Can you work these out from the model? Positions are in its coordinate system, mm. Coordinates: 2 decimals unless noted, no trailing zeros. Loops run counter-clockwise (first coordinate to the right, second up) from the corner with the lowest first, then second, coordinate; pieces in that order, holes last. Notation, with made-up numbers: M -23.5,-16.75 L 35.5,-16.75 A30 cw 35.5,8.25 Z; hole C 14.25,56.5 d11. An arc over 180 degrees is marked long. Return JSON: item names as keys, results as strings. Group by question number.
Autodesk Inventor part; units mm, degrees
ref_plane "YZ Plane" through (0, 0, 0) normal (1, 0, 0) x (0, 1, 0)
ref_plane "XZ Plane" through (0, 0, 0) normal (0, 1, 0) x (-1, 0, 0)
ref_plane "XY Plane" through (0, 0, 0) normal (0, 0, 1) x (1, 0, 0)
sketch "Sketch1" plane through (0, 0, 0) normal (1, 0, 0) x (0, 1, 0)
  line L0 (-50, 50) -> (50, 50)
  line L1 (50, 50) -> (50, -50)
  line L2 (50, -50) -> (-50, -50)
  line L3 (-50, -50) -> (-50, 50)
  line L4 (-50, 50) -> (50, -50) construction
  line L5 (50, 50) -> (-50, -50) construction
  line L6 (50, 50) -> (-50, 50)
  line L7 (-50, 50) -> (-50, 310)
  line L8 (-50, 310) -> (50, 310)
  line L9 (50, 310) -> (50, 50)
  line L10 (50, -50) -> (-50, -50)
  line L11 (-50, -50) -> (-50, -310)
  line L12 (-50, -310) -> (50, -310)
  line L13 (50, -310) -> (50, -50)
  line L14 (-50, 255) -> (-55, 255)
  line L15 (-55, 255) -> (-55, 205)
  line L16 (-55, 205) -> (-50, 205)
  line L17 (-50, 205) -> (-50, 255)
  line L18 (-50, 155) -> (-55, 155)
  line L19 (-55, 155) -> (-55, 105)
  line L20 (-55, 105) -> (-50, 105)
  line L21 (-50, 105) -> (-50, 155)
  line L22 (-50, 25) -> (-55, 25)
  line L23 (-55, 25) -> (-55, -25)
  line L24 (-55, -25) -> (-50, -25)
  line L25 (-50, -25) -> (-50, 25)
  line L26 (-50, -105) -> (-55, -105)
  line L27 (-55, -105) -> (-55, -155)
  line L28 (-55, -155) -> (-50, -155)
  line L29 (-50, -155) -> (-50, -105)
  line L30 (-50, -205) -> (-55, -205)
  line L31 (-55, -205) -> (-55, -255)
  line L32 (-55, -255) -> (-50, -255)
  line L33 (-50, -255) -> (-50, -205)
  line L34 (50, 310) -> (30, 310)
  line L35 (50, 305) -> (50, 310)
  line L36 (-50, 310) -> (-30, 310)
  line L37 (-50, 305) -> (-50, 310)
  line L38 (30, 50) -> (-30, 50)
  line L39 (-30, 50) -> (-30, 55)
  line L40 (-30, 55) -> (30, 55)
  line L41 (30, 55) -> (30, 50)
  line L42 (30, -50) -> (-36.1124, -50)
  line L43 (50, 0) -> (-50, 0) construction
  line L44 (-30, -50) -> (-30, -55)
  line L45 (-30, -55) -> (30, -55)
  line L46 (30, -55) -> (30, -50)
  line L47 (30, 310) -> (-30, 310)
  line L48 (-30, 310) -> (-30, 305)
  line L49 (-30, 305) -> (30, 305)
  line L50 (30, 305) -> (30, 310)
  line L51 (-30, -310) -> (-30, -305)
  line L52 (-30, -305) -> (30, -305)
  line L53 (30, -305) -> (30, -310)
  line L54 (-50, -180) -> (50, -180) construction
  circle A0 centre (0, -180) radius 16
  line L55 (50, 25) -> (45, 25)
  line L56 (45, 25) -> (45, -25)
  line L57 (45, -25) -> (50, -25)
  line L58 (50, -25) -> (50, 25)
  line L59 (50, -105) -> (45, -105)
  line L60 (45, -105) -> (45, -155)
  line L61 (45, -155) -> (50, -155)
  line L62 (50, -155) -> (50, -105)
  line L63 (50, -255) -> (45, -255)
  line L64 (45, -255) -> (45, -205)
  line L65 (45, -205) -> (50, -205)
  line L66 (-50, 11.5) -> (-32, 11.5)
  line L67 (-32, 11.5) -> (-32, -11.5)
  line L68 (-32, -11.5) -> (-50, -11.5)
  line L69 (-50, -11.5) -> (-50, 11.5)
  line L70 (-33.6603, 235) -> (-25, 240)
  line L71 (-25, 240) -> (-16.3397, 235)
  line L72 (-16.3397, 235) -> (-16.3397, 225)
  line L73 (-16.3397, 225) -> (-25, 220)
  line L74 (-25, 220) -> (-33.6603, 225)
  line L75 (-33.6603, 225) -> (-33.6603, 235)
  line L76 (-33.6603, 135) -> (-25, 140)
  line L77 (-25, 140) -> (-16.3397, 135)
  line L78 (-16.3397, 135) -> (-16.3397, 125)
  line L79 (-16.3397, 125) -> (-25, 120)
  line L80 (-25, 120) -> (-33.6603, 125)
  line L81 (-33.6603, 125) -> (-33.6603, 135)
  line L82 (-8.75, 225) -> (-13.75, 225)
  line L83 (-13.75, 225) -> (-13.75, 205)
  line L84 (-13.75, 205) -> (-8.75, 205)
  line L85 (-8.75, 205) -> (-8.75, 225)
  line L86 (-13.75, 135) -> (-8.75, 135)
  line L87 (-8.75, 135) -> (-8.75, 155)
  line L88 (-8.75, 155) -> (-13.75, 155)
  line L89 (-13.75, 155) -> (-13.75, 135)
  line L90 (-13.75, 85) -> (-8.75, 85)
  line L91 (-8.75, 85) -> (-8.75, 65)
  line L92 (-8.75, 65) -> (-13.75, 65)
  line L93 (-13.75, 65) -> (-13.75, 85)
  line L94 (-25, 314.14) -> (-25, -94.5604) construction
  line L95 (-41.25, 225) -> (-36.25, 225)
  line L96 (-36.25, 225) -> (-36.25, 205)
  line L97 (-36.25, 205) -> (-41.25, 205)
  line L98 (-41.25, 205) -> (-41.25, 225)
  line L99 (-36.25, 135) -> (-41.25, 135)
  line L100 (-41.25, 135) -> (-41.25, 155)
  line L101 (-41.25, 155) -> (-36.25, 155)
  line L102 (-36.25, 155) -> (-36.25, 135)
  line L103 (-36.25, 85) -> (-41.25, 85)
  line L104 (-41.25, 85) -> (-41.25, 65)
  line L105 (-41.25, 65) -> (-36.25, 65)
  line L106 (-36.25, 65) -> (-36.25, 85)
  line L107 (-15, 242.5) -> (-35, 242.5)
  line L108 (-35, 242.5) -> (-35, 247.5)
  line L109 (-35, 247.5) -> (-15, 247.5)
  line L110 (-15, 247.5) -> (-15, 242.5)
  line L111 (-15, 20) -> (-35, 20)
  line L112 (-35, 20) -> (-35, 25)
  line L113 (-35, 25) -> (-15, 25)
  line L114 (-15, 25) -> (-15, 20)
  line L115 (-20, 42.5) -> (-30, 42.5)
  line L116 (-30, 42.5) -> (-30, 32.5)
  line L117 (-30, 32.5) -> (-20, 32.5)
  line L118 (-20, 32.5) -> (-20, 42.5)
  point P0 (0, 0)
  point P1 (-52.5, 155)
  point P2 (-52.5, 205)
  point P3 (-50, 205)
  point P4 (-50, 105)
  point P5 (-50, -155)
  point P6 (-50, -255)
  point P7 (30, -50)
  point P8 (-30, -50)
  point P9 (-30, 50)
  point P10 (30, 50)
  point P11 (30, 307.5)
  point P12 (-30, -310)
  point P13 (30, -310)
  point P14 (30, 310)
  point P15 (-30, 310)
  point P16 (50, -25)
  point P17 (50, -255)
  point P18 (50, -205)
  point P19 (50, -155)
  point P20 (-50, 0)
  point P21 (-50, 11.5)
  point P22 (-50, -11.5)
  point P23 (-25, 230)
  point P24 (-25, 130)
  point P25 (-13.75, 145)
  point P26 (-36.25, 145)
  point P27 (-15, 22.5)
  point P28 (-30, 37.5)
  dimension "d0" = 100
  dimension "d1" = 260
  dimension "d2" = 100
  dimension "d3" = 260
  dimension "d4" = 50
  dimension "d5" = 50
  dimension "d6" = 50
  dimension "d7" = 50
  dimension "d8" = 50
  dimension "d9" = 55
  dimension "d10" = 50
  dimension "d11" = 25
  dimension "d12" = 55
  dimension "d13" = 50
  dimension "d14" = 5
  dimension "d20" = 5
  dimension "d21" = 5
  dimension "d23" = 20
  dimension "d26" = 32
  dimension "d27" = 5
  dimension "d28" = 5
  dimension "d29" = 18
  dimension "d30" = 23
  dimension "d31" = 11.5
  dimension "d32" = 20
  dimension "d34" = 10
  dimension "d35" = 25
  dimension "d37" = 25
  dimension "d38" = 16.3397
  dimension "d39" = 10
  dimension "d40" = 25
  dimension "d41" = 16.3397
  dimension "d42" = 25
  dimension "d43" = 11.25
  dimension "d44" = 20
  dimension "d45" = 0
  dimension "d46" = 5
  dimension "d47" = 20
  dimension "d48" = 5
  dimension "d49" = 11.25
  dimension "d50" = 50
  dimension "d51" = 20
  dimension "d52" = 5
  dimension "d53" = 11.25
  dimension "d54" = 11.25
  dimension "d55" = 20
  dimension "d56" = 10
  dimension "d57" = 5
  dimension "d58" = 12.5
  dimension "d59" = 5
  dimension "d60" = 20
  dimension "d61" = 10
  dimension "d62" = 40
  dimension "d63" = 10
  dimension "d64" = 10
  dimension "d65" = 5
  dimension "d66" = 7.5
extrude "Extrusion1" add sketch "Sketch1" along normal blind 5 contours L7 L8 L48 L49 L50 L9 L0 L41 L40 L39 | L0 L1 L55 L56 L57 L2 L3 L68 L67 L66 | L3 L24 L23 L22 | L20 L19 L18 L7 | L16 L15 L14 L7 | L2 L44 L45 L46 L13 L59 L60 L61 L65 L64 L63 L12 L53 L52 L51 L11 | L11 L28 L27 L26 | L11 L32 L31 L30
equation "\"BendRadius\" = Thickness"
equation "\"BendReliefWidth\" = Thickness"
equation "\"BendReliefDepth\" = 0.5 * Thickness"
equation "\"CornerReliefSize\" = 4 * Thickness"
equation "\"MinimumRemnant\" = 2 * Thickness"
equation "\"TransitionRadius\" = BendRadius"
equation "\"JacobiRadiusSize\" = BendRadius"
equation "\"GapSize\" = Thickness"
properties part number "Lat2" material "Wood (Cherry)"
1) Suppose I cut it at D-D, the plane z = -75.5. List the corners of the cut face in (x, y) for me, then the cut area to 3 significant figures.
2) Suppose I cut it at A-A, the plane y = 0. List the corners of the cut face in (x, z) for me, then the cut area to 3 significant figures.
3) Suppose I cut it at C-C, the plane x = 1.9. Give the number of separate pieces and of enclosed holes in the cut face, then the cut area to 3 significant figures.
4) If we mould it in two halves opening along Y, with no side actions, what happens to faces 1 (the face through (2.465, 7.383, -165.805)), 2 (the face through (0, -3, 4))? For each: +Y half, -Y half, draft (parallel to the pull), parting line (faces both ways), or undercut.
5) If I drill on line 1 (Z direction, x = 1.9, y = 46); line 2 (Z direction, x = 3.15, y = 0); line 3 (Z direction, x = 0.9, y = -40.5), over which ranges is the centre line in solid material (lowest first)? Write a range as from..to.
6) For pin 1 (1.5 mm diameter, centred on x = 1.5, z = 51.5, fed in from -Y); pin 2 (1.5 mm diameter, centred on x = 2.5, y = -25.5, fed in from -Z); pin 3 (1.5 mm diameter, centred on x = 2, y = -53.5, fed in from +Z), each with a flat end and sliding along its axis, tell me the tip position at first contact or that it passes through.
7) Suppose I cut it at B-B, the plane z = -180. List the corners of the cut face in (x, y) for me.
Returned:
{
 "1": {"outline": "M 0,-50 L 5,-50 L 5,50 L 0,50 Z", "area": "500 mm²"},
 "2": {"outline": "M 0,-305 L 5,-305 L 5,-196 L 0,-196 Z; M 0,-164 L 5,-164 L 5,-55 L 0,-55 Z; M 0,-50 L 5,-50 L 5,50 L 0,50 Z; M 0,55 L 5,55 L 5,305 L 0,305 Z", "area": "2,840 mm²"},
 "3": {"separate pieces": "1", "enclosed holes": "15", "area": "58,700 mm²"},
 "4": {"face 1": "undercut", "face 2": "draft"},
 "5": {"line 1": "z = -310..-255, -205..-155, -105..-25, 25..310", "line 2": "z = -305..-196, -164..-55, -50..50, 55..305", "line 3": "z = -310..-11.5, 11.5..65, 85..135, 155..205, 225..310"},
 "6": {"pin 1": "stops at y = -50", "pin 2": "stops at z = -305", "pin 3": "stops at z = 255"},
 "7": {"outline": "M 0,-50 L 5,-50 L 5,-16 L 0,-16 Z; M 0,16 L 5,16 L 5,50 L 0,50 Z"}
}
